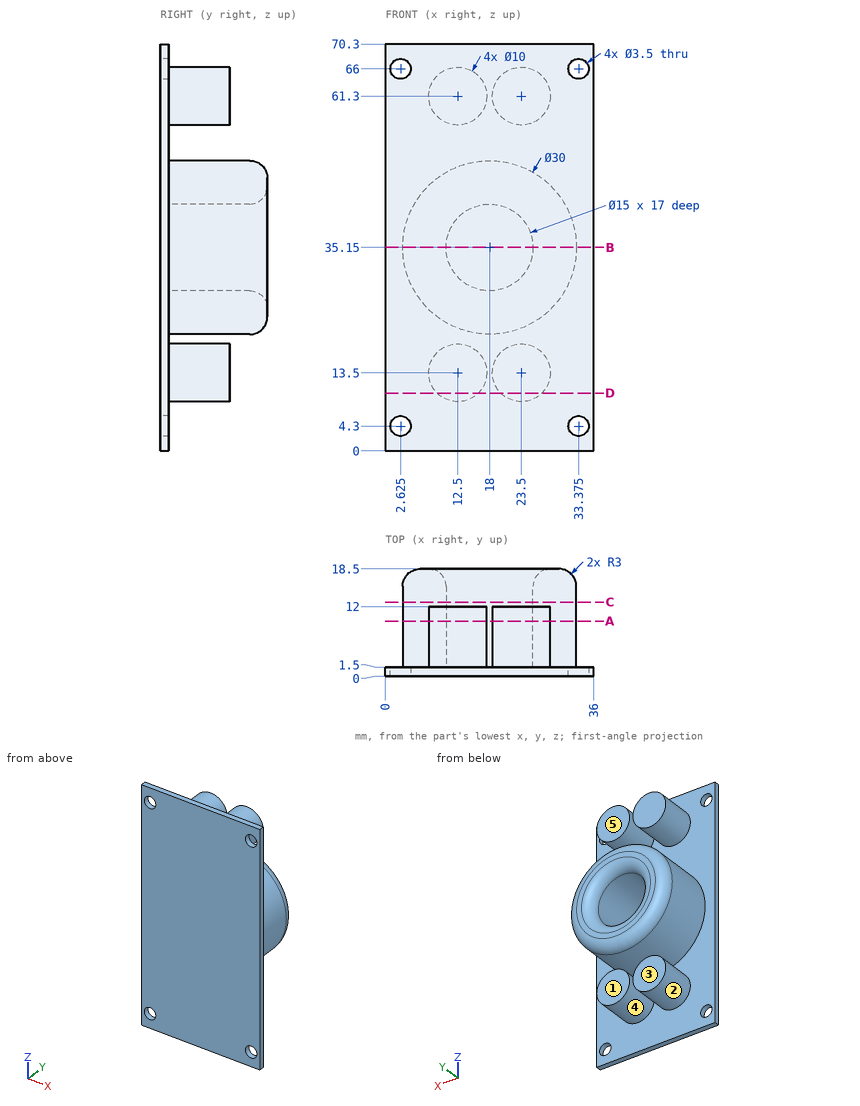
Answer from the drawing. Dimensions are ordinates in mm from the lowest x, y and z of the part. A direction names the side the tool comes from. Give positions to 0.01 mm unless a question says otherwise; leave off trailing zeros. Write each loop counter-clockwise with the first axis right and the second up, starting at its lowest first coordinate (ties: lowest second). Pieces come first, ordered by that corner, then holes. Notation, with made-up numbers: (46.5, 48.5) -> (63.5, 48.5) arc R19 ccw to (63.5, 53.5) -> close; hole circle Ø5 at (53, 53.5). An arc over 180 degrees is marked (long way). One line per question, with ' | ' between items. Start each with the question number.
1. For the marked faces 3, 4 and 5, determine the directions among +Z, -Z, +X, -X, +Y, -Y from which every point of the face is accessible in a straight line to the end or side of a thin tool.
2. Given pin 1 Ø2 at (x, z) = (2.625, 4.3) entering from +Y; pin 2 Ø4 at (y, z) = (10, 20.5) entering from +X; pin 3 Ø4 at (y, z) = (12.5, 32.5) entering from +X; pin 4 Ø3 at (x, z) = (11, 12) entering from +Y, each flat-ended and moving along its own axis, determine where each tip first touches the part or whether it passes through.
3. Find the intervals of material crossed by probe 1 along X at (y, z) = (0.5, 66) (3 decimals); probe 2 along Z at (x, y) = (18, 12); probe 3 along Y at (x, z) = (23.5, 4.5), in increasing order.
4. Section C-C (y = 12.75) is taken. Determine the outline of the cut face in (x, z).
5. Section B-B (z = 35.15) is taken. Determine the outline of the cut face in (x, y), plus the area to 3 significant figures.
6. Section D-D (z = 10) is taken. Determine the outline of the cut face in (x, y).
7. For a pull along Z with two mould halves and no side action, classify the marked faces 1 and 2 as pulls with the +Z half, pulls with the -Z half, needs draft (parallel to the pull), parting line crosses it, or undercut.
8. Section A-A (y = 9.5) is taken. Determine the outline of the cut face in (x, z).
Response values:
1) face 3: -Z, +X, -X, +Y | face 4: +Y | face 5: +Z, +X, -X, +Y
2) pin 1: through | pin 2: x = 26.06 | pin 3: x = 32.99 | pin 4: y = 12
3) probe 1: 0 to 0.875, 4.375 to 31.625, 35.125 to 36 | probe 2: 20.15 to 27.65, 42.65 to 50.15 | probe 3: 0 to 1.5
4) outline: circle Ø30 at (18, 35.15); hole circle Ø15 at (18, 35.15)
5) outline: (0, 0) -> (36, 0) -> (36, 1.5) -> (33, 1.5) -> (33, 15.5) arc R3 ccw to (30, 18.5) -> (28.5, 18.5) arc R3 ccw to (25.5, 15.5) -> (25.5, 1.5) -> (10.5, 1.5) -> (10.5, 15.5) arc R3 ccw to (7.5, 18.5) -> (6, 18.5) arc R3 ccw to (3, 15.5) -> (3, 1.5) -> (0, 1.5) -> close | area: 301 mm2
6) outline: (0, 0) -> (36, 0) -> (36, 1.5) -> (27.07, 1.5) -> (27.07, 12) -> (19.93, 12) -> (19.93, 1.5) -> (16.07, 1.5) -> (16.07, 12) -> (8.93, 12) -> (8.93, 1.5) -> (0, 1.5) -> close
7) face 1: needs draft | face 2: undercut
8) outline: circle Ø30 at (18, 35.15); circle Ø10 at (12.5, 13.5); circle Ø10 at (12.5, 61.3); circle Ø10 at (23.5, 13.5); circle Ø10 at (23.5, 61.3); hole circle Ø15 at (18, 35.15)
